from build123d import *

# Parameters (mm, degrees)
SKETCH2_W           = 10
SKETCH2_H           = 50
BOSS_EXTRUDE1_DEPTH = 10
SKETCH6_R           = 2.65
CUT_EXTRUDE3_DEPTH  = 11
SKETCH7_R           = 2.35
SKETCH7_R_2         = 2.65
CUT_EXTRUDE4_DEPTH  = 11
SKETCH8_W           = 1.5
SKETCH8_H           = 21
BOSS_EXTRUDE2_DEPTH = 30
SKETCH9_W           = 52.99414334
SKETCH9_H           = 19.059793282
CUT_EXTRUDE5_DEPTH  = 11


with BuildPart() as part:
    # Sketch2 → Boss-Extrude1 (new body)
    with BuildSketch(Plane.XY):
        with Locations((5, 25)):
            Rectangle(SKETCH2_W, SKETCH2_H)
    extrude(amount=BOSS_EXTRUDE1_DEPTH)

    # Sketch6 → Cut-Extrude3 (cut, through all)
    with BuildSketch(Plane.XY.offset(10)):
        with Locations((5, 27)):
            Circle(SKETCH6_R)
    extrude(amount=-CUT_EXTRUDE3_DEPTH, mode=Mode.SUBTRACT)

    # Sketch7 → Cut-Extrude4 (cut, through all)
    with BuildSketch(Plane.ZY):
        with Locations((5, 41)):
            Circle(SKETCH7_R)
        with Locations((5, 9)):
            Circle(SKETCH7_R_2)
    extrude(amount=-CUT_EXTRUDE4_DEPTH, mode=Mode.SUBTRACT)

    # Sketch8 → Boss-Extrude2 (add)
    with BuildSketch(Plane.ZY):
        with Locations((9.25, 26)):
            Rectangle(SKETCH8_W, SKETCH8_H)
        with Locations((0.75, 26)):
            Rectangle(SKETCH8_W, SKETCH8_H)
    extrude(amount=BOSS_EXTRUDE2_DEPTH)

    # Sketch9 → Cut-Extrude5 (cut, through all)
    with BuildSketch(Plane.XY.offset(10)):
        with Locations((-7.642110933, 41.529896641)):
            Rectangle(SKETCH9_W, SKETCH9_H)
    extrude(amount=-CUT_EXTRUDE5_DEPTH, mode=Mode.SUBTRACT)


solid = part.part
Here's how the part is built. I have some questions about the finished solid (model axes, mm). A direction names the side the tool comes from. Give positions to 0.01 mm unless a question says otherwise; leave off trailing zeros. Order: outer loops, then holes, each group sorted by start corner. A loop starts at its lowest first (then second) coordinate and runs counter-clockwise, first axis right, second up. Notation, with made-up numbers: (40, -13) -> (71, -13) arc R12 ccw to (71, 1) -> close; hole circle Ø5 at (88.25, 16.25). An arc over 180 degrees is marked (long way). One line per item, written item: value. Start each with the question number.
1. Will these pins go through, and if not, where does the flat tip stop? pin 1 Ø5 at (x, z) = (-12, 5) entering from -Y; pin 2 Ø6 at (x, z) = (-14, 2.5) entering from -Y.
2. Imagine slicing it at C-C, the plane y = 27. List the corners of the cut face in (x, z) for me.
3. I need wall thicknesses on probe 1 along Z at (x, y) = (-28, 16.5); probe 2 along Y at (x, z) = (-1, 9.25); probe 3 along X at (y, z) = (18.5, 7.75). Which ranges of each line are inside material? Lowest first, please. Write a range as from..to.
4. Imagine slicing it at D-D, the plane x = -5. List the corners of the cut face in (y, z) for me, plus the area to 3 significant figures.
5. For faces 5 (the face through (-15, 24, 1.5)), 6 (the face through (-15, 15.5, 9)), 7 (the face through (6.223, 24.649, 5.07)), which set-ups out of +Z, -Z, +X, -X, +Y, -Y let a thin tool reach every point of the face, with its end or its side?
6. Imagine slicing it at A-A, the plane x = 5. List the corners of the cut face in (y, z) for me.
7. We'd pull the mould along Z, two halves only. Please class faces 1 (the face through (-10, 20, 0)), 2 (the face through (4.93, 6.649, 6.223)), 3 (the face through (-15, 15.5, 1)), 4 (the face through (-10, 20, 10)): released by +Z, released by -Z, zero draft, split by the parting line, or undercut.
8. Imagine slicing it at B-B, the plane z = 5. List the corners of the cut face in (x, y) for me, plus the area to 3 significant figures.
Values follow:
1. pin 1: passes through
1. pin 2: stops at y = 15.5
2. outline: (-30, 0) -> (2.35, 0) -> (2.35, 10) -> (-30, 10) -> (-30, 8.5) -> (0, 8.5) -> (0, 1.5) -> (-30, 1.5) -> close; (7.65, 0) -> (10, 0) -> (10, 10) -> (7.65, 10) -> close
3. probe 1: z = 0..1.5, 8.5..10
3. probe 2: y = 15.5..32
3. probe 3: x = 0..10
4. outline: (15.5, 0) -> (32, 0) -> (32, 1.5) -> (15.5, 1.5) -> close; (15.5, 8.5) -> (32, 8.5) -> (32, 10) -> (15.5, 10) -> close
4. area: 49.5 mm2
5. face 5: -X, +Y, -Y
5. face 6: +Z, -Z, -X, -Y
5. face 7: +Z, -Z
6. outline: (0, 0) -> (24.35, 0) -> (24.35, 10) -> (0, 10) -> close; (29.65, 0) -> (32, 0) -> (32, 10) -> (29.65, 10) -> close; hole circle Ø5.3 at (9, 5)
7. face 1: released by -Z
7. face 2: undercut
7. face 3: zero draft
7. face 4: released by +Z
8. outline: (0, 0) -> (10, 0) -> (10, 6.35) -> (0, 6.35) -> close; (0, 11.65) -> (10, 11.65) -> (10, 32) -> (0, 32) -> close; hole circle Ø5.3 at (5, 27)
8. area: 245 mm2
